```python
from build123d import *

# Parameters (mm, degrees)
SKETCH1_W          = 72.39
SKETCH1_H          = 12.7
BASE_FLANGE1_DEPTH = 0.91186
EDGE_FLANGE1_DEPTH = 12.7
EDGE_FLANGE2_DEPTH = 12.7
EDGE_FLANGE3_DEPTH = 12.7
EDGE_FLANGE4_DEPTH = 72.39


# Sheet-metal steps are written as plain solids
with BuildPart() as part:
    # Sketch1 → Base-Flange1 (new body)
    with BuildSketch(Plane(origin=(0, 0, 0), x_dir=(1, 0, 0), z_dir=(0, 1, 0))):
        with Locations((36.195, 6.35)):
            Rectangle(SKETCH1_W, SKETCH1_H)
    extrude(amount=-BASE_FLANGE1_DEPTH)

    # Edge-Flange1 section (across the edge) → Edge-Flange1 (add)
    with BuildSketch(Plane(origin=(-1.27, -0.91186, 0), x_dir=(1, 0, 0), z_dir=(0, 0, -1))):
        with BuildLine():
            Line((-0.91186, 1.27), (-0.91186, 19.40814))
            Line((-0.91186, 19.40814), (0, 19.40814))
            Line((0, 19.40814), (0, 1.27))
            ThreePointArc((0, 1.27), (0.371974388, 0.371974388), (1.27, 0))
            Line((1.27, 0), (1.27, -0.91186))
            ThreePointArc((1.27, -0.91186), (-0.272808002, -0.272808002), (-0.91186, 1.27))
        make_face()
    extrude(amount=EDGE_FLANGE1_DEPTH)

    # Edge-Flange2 section (across the edge) → Edge-Flange2 (add)
    with BuildSketch(Plane(origin=(73.66, -0.91186, -12.7), x_dir=(-1, 0, 0), z_dir=(0, 0, 1))):
        with BuildLine():
            Line((-0.91186, 1.27), (-0.91186, 5.43814))
            Line((-0.91186, 5.43814), (0, 5.43814))
            Line((0, 5.43814), (0, 1.27))
            ThreePointArc((0, 1.27), (0.371974388, 0.371974388), (1.27, 0))
            Line((1.27, 0), (1.27, -0.91186))
            ThreePointArc((1.27, -0.91186), (-0.272808002, -0.272808002), (-0.91186, 1.27))
        make_face()
    extrude(amount=EDGE_FLANGE2_DEPTH)

    # Edge-Flange3 section (across the edge) → Edge-Flange3 (add)
    with BuildSketch(Plane(origin=(74.57186, -7.62, 0), x_dir=(0, 1, 0), z_dir=(0, 0, -1))):
        with BuildLine():
            Line((-0.91186, 1.27), (-0.91186, 10.51814))
            Line((-0.91186, 10.51814), (0, 10.51814))
            Line((0, 10.51814), (0, 1.27))
            ThreePointArc((0, 1.27), (0.371974388, 0.371974388), (1.27, 0))
            Line((1.27, 0), (1.27, -0.91186))
            ThreePointArc((1.27, -0.91186), (-0.272808002, -0.272808002), (-0.91186, 1.27))
        make_face()
    extrude(amount=EDGE_FLANGE3_DEPTH)

    # Edge-Flange4 section (across the edge) → Edge-Flange4 (add)
    with BuildSketch(Plane(origin=(0, -0.91186, -13.97), x_dir=(0, 0, 1), z_dir=(1, 0, 0))):
        with BuildLine():
            Line((-0.91186, 1.27), (-0.91186, 5.43814))
            Line((-0.91186, 5.43814), (0, 5.43814))
            Line((0, 5.43814), (0, 1.27))
            ThreePointArc((0, 1.27), (0.371974388, 0.371974388), (1.27, 0))
            Line((1.27, 0), (1.27, -0.91186))
            ThreePointArc((1.27, -0.91186), (-0.272808002, -0.272808002), (-0.91186, 1.27))
        make_face()
    extrude(amount=EDGE_FLANGE4_DEPTH)


solid = part.part
```
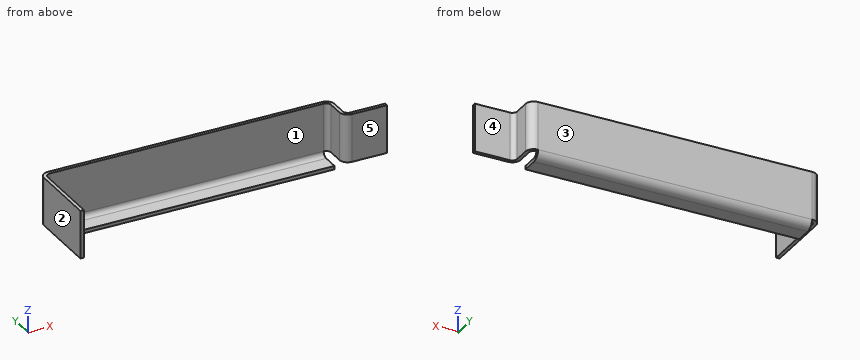
For this review, take the finished solid that the model builds, in its own axes (mm). Face numbers are marked on the shaded views. A direction names the side the tool comes from. Give positions to 0.01 mm unless a question says otherwise; leave off trailing zeros. Order: outer loops, then holes, each group sorted by start corner. A loop starts at its lowest first (then second) coordinate and runs counter-clockwise, first axis right, second up.
1) Take a section at C-C (y = -14.5). Give the boundary of the cut face in (x, z), then the cut area to 3 significant figures.
2) Take a section at A-A (x = 47). Give the boundary of the cut face in (y, z).
3) Wall thickness on line 1 (Y direction, x = 54, z = -9.25); line 2 (X direction, y = -15.75, z = -4); line 3 (X direction, y = -2.5, z = -1): over which ranges is each line inside the solid? List them lowest first.
4) Take a section at B-B (z = -11). Give the boundary of the cut face in (x, y), then the cut area to 3 significant figures.
5) Insertion check: pin 1 (2 mm diameter, centred on y = -17.5, z = -9, fed in from +X); pin 2 (4.5 mm diameter, centred on x = 80.5, z = -4, fed in from +Y); pin 3 (2 mm diameter, centred on y = -5, z = -7, fed in from +X); pin 4 (4 mm diameter, centred on y = -11, z = -13.5, fed in from -X). Each pin has a flat end and moves straight along its axis. Give the tip position at first contact, or say it passes through.
6) For the marked faces 4 and 5, list the 3-axis set-ups (+Z, -Z, +X, -X, +Y, -Y) from which the entire face can be reached by the end or side of a thin tool; tool diameter is ignored.
7) The part is to be moulded in two halves that separate along X. For the marked faces 1, 2 and 3, say which applies: released by +X, released by -X, zero draft, split by the parting line, or undercut.
Derived:
1. outline: (-2.18, -12.7) - (-1.27, -12.7) - (-1.27, 0) - (-2.18, 0) - close
1. area: 11.6 mm2
2. outline: (-6.35, -14.88) - (-2.18, -14.88) arc R2.18 ccw to (0, -12.7) - (0, 0) - (-0.91, 0) - (-0.91, -12.7) arc R1.27 cw to (-2.18, -13.97) - (-6.35, -13.97) - close
3. line 1: y = -0.91 to 0
3. line 2: x = -2.18 to -1.27
3. line 3: x = -2.18 to -1.27, 73.66 to 74.57
4. outline: (-2.18, -20.32) - (-1.27, -20.32) - (-1.27, -2.18) arc R1.27 cw to (0, -0.91) - (72.39, -0.91) arc R1.27 cw to (73.66, -2.18) - (73.66, -6.35) arc R2.18 ccw to (75.84, -8.53) - (85.09, -8.53) - (85.09, -7.62) - (75.84, -7.62) arc R1.27 cw to (74.57, -6.35) - (74.57, -2.18) arc R2.18 ccw to (72.39, 0) - (0, 0) arc R2.18 ccw to (-2.18, -2.18) - close
4. area: 102 mm2
5. pin 1: stops at x = -1.27
5. pin 2: stops at y = -7.62
5. pin 3: stops at x = 74.57
5. pin 4: stops at x = -2.18
6. face 4: +Z, -Z, +X, +Y
6. face 5: +Z, -Z, +X, -Y
7. face 1: undercut
7. face 2: released by -X
7. face 3: zero draft
